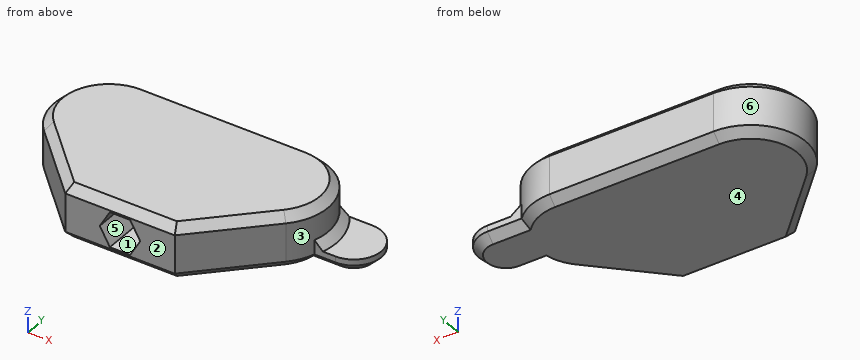
Autodesk Fusion 360 part; units mm, degrees
sketch "Sketch1" plane through (0, 0, 0) normal (0, 0, 1) x (1, 0, 0)
  line L0 (-10, 0) -> (10, 0)
  line L1 (10, 0) -> (22.0711, 12.0711)
  arc A0 (22.0711, 12.0711) -> (15, 29.1421) centre (15, 19.1421) ccw
  line L2 (15, 29.1421) -> (-15, 29.1421)
  arc A1 (-15, 29.1421) -> (-22.0711, 12.0711) centre (-15, 19.1421) ccw
  line L3 (-22.0711, 12.0711) -> (-10, 0)
  line L4 (0, 0) -> (0, 29.1421) construction
  line L5 (-24, 23.501) -> (-24, 41.501)
  line L6 (-24, 41.501) -> (-18, 41.501)
  line L7 (-18, 41.501) -> (-18, 28.6815)
  line L8 (22.1414, 26.1421) -> (28.351, 26.1421)
  arc A2 (28.351, 16.1421) -> (28.351, 26.1421) centre (28.351, 21.1421) ccw
  line L9 (28.351, 16.1421) -> (24.5394, 16.1421)
  dimension "d1" = 10
  dimension "d2" = 135
  dimension "d3" = 50
  dimension "d4" = 20
  dimension "d5" = 6
  dimension "d6" = 18
  dimension "d7" = 18
  dimension "d18" = 5
  dimension "d19" = 3
  dimension "d20" = 3.5
extrude "Extrude1" add sketch "Sketch1" along normal mid plane 10 contours L0 L1 A0 L2 A1 L3
extrude "Extrude3" add sketch "Sketch1" along normal blind 2.6 from surface at -5 contours A0 L8 A2 L9
sketch "Sketch2" plane through (0, 0, 0) normal (0, 1, 0) x (1, 0, 0)
  line L0 (3.695, 0) -> (1.8475, 3.2)
  line L1 (1.8475, 3.2) -> (-1.8475, 3.2)
  line L2 (-1.8475, 3.2) -> (-3.695, 0)
  line L3 (-3.695, 0) -> (-1.8475, -3.2)
  line L4 (-1.8475, -3.2) -> (1.8475, -3.2)
  line L5 (1.8475, -3.2) -> (3.695, 0)
  dimension "d10" = 6.4
extrude "Extrude2" cut sketch "Sketch2" along normal blind 16
chamfer "Chamfer1" distance 1.5 angle 45 1 edges at (24.7243, 21.474, -2.4) 2 faces at (3.3333, 19.4281, 5) (3.3333, 19.4281, -5)
The model under review builds one solid part; all positions refer to its coordinate system, in mm. Face numbers are marked on the shaded views. A direction names the side the tool comes from. Give positions to 0.01 mm unless a question says otherwise; leave off trailing zeros. Loops run counter-clockwise (first coordinate to the right, second up) from the corner with the lowest first, then second, coordinate; pieces in that order, holes last. Notation, with made-up numbers: (32.5, 9) - (42.5, 9) arc R37 ccw to (42.5, 45) - close; hole circle Ø7 at (-7, -15). An arc over 180 degrees is marked (long way). Answer as a JSON object with one key per item and string values.
Q1. Insertion check: pin 1 (3 mm diameter, centred on x = 26, z = -2.5, fed in from +Y); pin 2 (3 mm diameter, centred on x = 27, z = -1.5, fed in from -Y); pin 3 (7.5 mm diameter, centred on x = 27.5, y = 21, fed in from +Z). Each pin has a flat end and moves straight along its axis. Give the tip position at first contact, or say it passes through.
Worked out:
{"pin 1": "stops at y = 26.14", "pin 2": "stops at y = 16.14", "pin 3": "stops at z = 4.61"}
Q2. Add section C-C on x = -11.5. State the section outline as (y, z) points.
Worked out:
{"outline": "(1.5, -3.5) - (3.62, -5) - (27.64, -5) - (29.14, -3.5) - (29.14, 3.5) - (27.64, 5) - (3.62, 5) - (1.5, 3.5) - close"}
Q3. Mouldability with a two-part tool opening along X and no side actions: class the marked faces 4, 5 and 6 as +X half, -X half, draft (parallel to the pull), parting line (faces both ways), or undercut.
Worked out:
{"face 4": "draft", "face 5": "undercut", "face 6": "-X half"}
Q4. To check wall thickness, follow line 1 along X through (y, z) = (19, -0.75); line 2 along X through (y, z) = (6.5, 1.25); line 3 along Y through (x, z) = (-15, -1). State the ranges of each line that lie inside material, in increasing order.
Worked out:
{"line 1": "x = -25 to 25", "line 2": "x = -16.5 to -2.97, 2.97 to 16.5", "line 3": "y = 5 to 29.14"}
Q5. For the marked faces 1, 2 and 3, list the 3-axis set-ups (+Z, -Z, +X, -X, +Y, -Y) from which the entire face can be reached by the end or side of a thin tool; tool diameter is ignored.
Worked out:
{"face 1": "-Y", "face 2": "+Z, -Z, +X, -X, -Y", "face 3": "+Z, +X"}
Q6. Add section B-B on z = -1.5. State the section outline as (x, y) points.
Worked out:
{"outline": "(-22.07, 12.07) - (-10, 0) - (-2.83, 0) - (-2.83, 16) - (2.83, 16) - (2.83, 0) - (10, 0) - (22.07, 12.07) arc R10 ccw to (24.54, 16.14) - (25.17, 16.14) arc R10.6 ccw to (22.96, 26.14) - (22.14, 26.14) arc R10 ccw to (15, 29.14) - (-15, 29.14) arc R10 ccw to start"}
Q7. Add section A-A on y = 8.5. State the section outline as (x, z) points (1 decimal).
Worked out:
{"outline": "(-18.5, -3.5) - (-16.4, -5) - (16.4, -5) - (18.5, -3.5) - (18.5, 3.5) - (16.4, 5) - (-16.4, 5) - (-18.5, 3.5) - close; hole (-3.7, 0) - (-1.8, -3.2) - (1.8, -3.2) - (3.7, 0) - (1.8, 3.2) - (-1.8, 3.2) - close"}
